CAD build for the part. Positions are in the model's coordinates, mm. Face numbers are marked on the shaded views. Give positions to 0.01 mm unless a question says otherwise; leave off trailing zeros. Write each loop counter-clockwise with the first axis right and the second up, starting at its lowest first coordinate (ties: lowest second). Pieces come first, ordered by that corner, then holes. Notation, with made-up numbers: (-5, -31) - (18, -31) arc R12 ccw to (18, -14) - close; hole circle Ø9 at (15.5, 69). An arc over 180 degrees is marked (long way). Answer as a JSON object with one key per item and string values.
from build123d import *

# Parameters (mm, degrees)
BOSS_EXTRUDE1_DEPTH = 6
SKETCH2_R           = 2.804848486
CUT_EXTRUDE1_DEPTH  = 3


with BuildPart() as part:
    # Sketch1 → Boss-Extrude1 (new body)
    with BuildSketch(Plane(origin=(0, 0, 0), x_dir=(0, 1, 0), z_dir=(0, 0, 1))):
        with BuildLine():
            Line((0, 5), (25, 5))
            ThreePointArc((25, 5), (25.828163089, 4.930937629), (26.633448216, 4.725658359))
            Line((26.633448216, 4.725658359), (64.438715088, -8.341927368))
            ThreePointArc((64.438715088, -8.341927368), (71.86918023, -46.91040032), (50.641475986, -13.863108592))
            Line((50.641475986, -13.863108592), (25, -5))
            Line((25, -5), (0, -5))
            ThreePointArc((0, -5), (-5, 0), (0, 5))
        make_face()
    extrude(amount=BOSS_EXTRUDE1_DEPTH)

    # Sketch2 → Cut-Extrude1 (cut)
    with BuildSketch(Plane(origin=(0, 0, 0), x_dir=(1, 0, 0), z_dir=(0, 0, -1))):
        with Locations(Location((0, 0, 0), (0, 0, 180))):
            Circle(SKETCH2_R)
    extrude(amount=-CUT_EXTRUDE1_DEPTH, mode=Mode.SUBTRACT)


solid = part.part
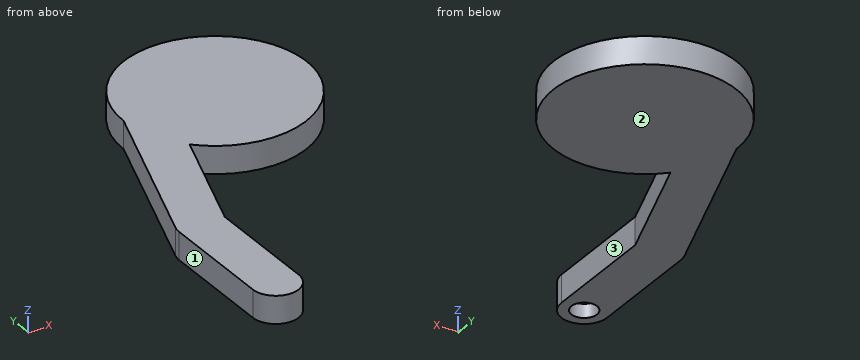
(1) Saw through at B-B, the plane x = 0. Give the cut face in (y, z), and give its area (3 significant figures).
Answer key:
{"outline": "(-5, 0) - (-2.8, 0) - (-2.8, 3) - (2.8, 3) - (2.8, 0) - (40.31, 0) - (40.31, 6) - (-5, 6) - close", "area": "255 mm²"}
(2) Saw through at C-C, the plane y = 17.5. Give the cut face in (x, z), and give its area (3 significant figures).
Answer key:
{"outline": "(-5, 0) - (5, 0) - (5, 6) - (-5, 6) - close", "area": "60.0 mm²"}
(3) Flat gauge pins, fed straight in: P1, Ø1.7, axis at x = 0, y = -1, coming from the -Z side; P2, Ø1.5, axis at x = 37, z = 1, coming from the -Y side. Where does each tip first touch, or does it go through?
Answer key:
{"P1": "stops at z = 3", "P2": "stops at y = 46.07"}
(4) Pull direction X, two halves, no side cores. Call the marked faces 1, 2 and 3: pulls with the +X half, pulls with the -X half, needs draft (parallel to the pull), parting line crosses it, or undercut.
Answer key:
{"face 1": "pulls with the -X half", "face 2": "needs draft", "face 3": "pulls with the +X half"}
(5) Saw through at A-A, the plane z = 0.9. Give the cut face in (x, y), and give its area (3 significant figures).
Answer key:
{"outline": "(-5, 0) arc R5 ccw to (5, 0) - (5, 25) - (13.86, 50.64) arc R20 ccw (long way) to (8.34, 64.44) - (-4.73, 26.63) arc R5 ccw to (-5, 25) - close; hole circle Ø5.61 at (0, 0)", "area": "1,840 mm²"}
(6) Probe L1, parallel to X at y = 9.5, z = 2.7; L2, parallel to X at y = 79, z = 4.15; L3, parallel to Y at x = 44, z = 5.5. List the from-to ranges inside material, lowest first. Write a range as [from, to].
Answer key:
{"L1": "x = [-5, 5]", "L2": "x = [14.63, 42.05]", "L3": "y = [52, 76.88]"}
(7) Saw through at D-D, the plane y = 77.5. Give the cut face in (x, z).
Answer key:
{"outline": "(13.2, 0) - (43.49, 0) - (43.49, 6) - (13.2, 6) - close"}
